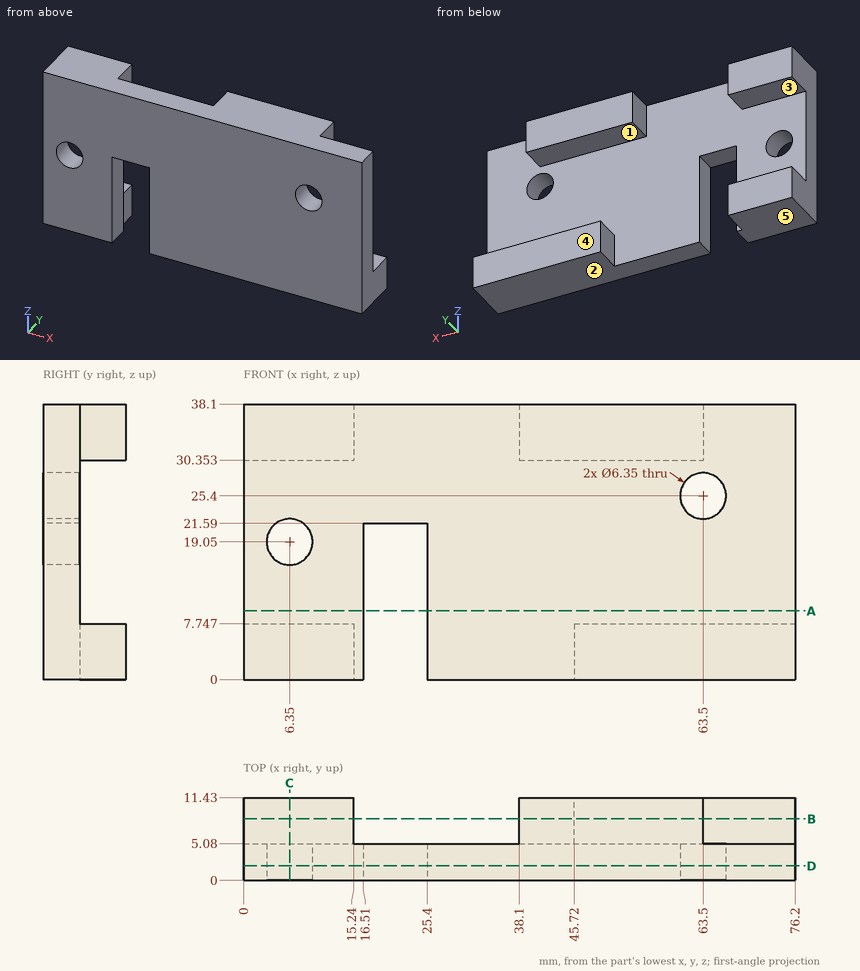
Answer from the drawing. Dimensions are ordinates in mm from the lowest x, y and z of the part. A direction names the side the tool comes from. Give positions to 0.01 mm unless a question says otherwise; leave off trailing zeros. Write each loop counter-clockwise with the first axis right and the second up, starting at its lowest first coordinate (ties: lowest second). Pieces come first, ordered by that corner, then holes. Notation, with made-up numbers: (53.25, 12) -> (62.25, 12) arc R22 ccw to (62.25, 46) -> close; hole circle Ø5 at (-23, 31.5). An arc over 180 degrees is marked (long way). Use a Markdown table: item, result.
(1) Determine the mould class of the marked faces 3, 4 and 5 for opening direction Z: released by +Z, released by -Z, zero draft, split by the parting line, or undercut.
Return value:
| item | result |
|---|---|
| face 3 | undercut |
| face 4 | zero draft |
| face 5 | released by -Z |
(2) Section A-A, the plane z = 9.5 is taken. Determine the outline of the cut face in (x, y), then the cut area to 3 significant figures.
Return value:
| item | result |
|---|---|
| outline | (0, 0) -> (16.51, 0) -> (16.51, 5.08) -> (0, 5.08) -> close; (25.4, 0) -> (76.2, 0) -> (76.2, 5.08) -> (25.4, 5.08) -> close |
| area | 342 mm2 |
(3) Find the intervals of material crossed by probe 1 along Z at (x, y) = (6.35, 1.3) (3 decimals); probe 2 along Z at (x, y) = (56.5, 8.75); probe 3 along X at (y, z) = (4.75, 7.5), in increasing order. Write a range as from..to.
Return value:
| item | result |
|---|---|
| probe 1 | 0..15.875, 22.225..38.1 |
| probe 2 | 0..7.75, 30.35..38.1 |
| probe 3 | 0..16.51, 25.4..76.2 |
(4) Flat-ended cylindrical pins translate along their axes: P1, Ø12, axis at x = 7.5, z = 19.5, coming from the +Y side; P2, Ø3, axis at y = 9, z = 35.5, coming from the +X side. Find the tip coordinate at first contact, or state that the pin passes through.
Return value:
| item | result |
|---|---|
| P1 | y = 5.08 |
| P2 | x = 63.5 |
(5) For the marked faces 1 and 2, determine the directions among +Z, -Z, +X, -X, +Y, -Y from which every point of the face is accessible in a straight line to the end or side of a thin tool.
Return value:
| item | result |
|---|---|
| face 1 | +X, -X, +Y |
| face 2 | -Z, +X, -X, +Y, -Y |
(6) Section D-D, the plane y = 2 is taken. Determine the outline of the cut face in (x, z) (3 decimals).
Return value:
| item | result |
|---|---|
| outline | (0, 0) -> (16.51, 0) -> (16.51, 21.59) -> (25.4, 21.59) -> (25.4, 0) -> (76.2, 0) -> (76.2, 38.1) -> (0, 38.1) -> close; hole circle Ø6.35 at (6.35, 19.05); hole circle Ø6.35 at (63.5, 25.4) |
(7) Section C-C, the plane x = 6.35 is taken. Determine the outline of the cut face in (y, z) (3 decimals).
Return value:
| item | result |
|---|---|
| outline | (0, 0) -> (11.43, 0) -> (11.43, 7.747) -> (5.08, 7.747) -> (5.08, 15.875) -> (0, 15.875) -> close; (0, 22.225) -> (5.08, 22.225) -> (5.08, 30.353) -> (11.43, 30.353) -> (11.43, 38.1) -> (0, 38.1) -> close |
(8) Section B-B, the plane y = 8.5 is taken. Determine the outline of the cut face in (x, z).
Return value:
| item | result |
|---|---|
| outline | (0, 0) -> (15.24, 0) -> (15.24, 7.75) -> (0, 7.75) -> close; (0, 30.35) -> (15.24, 30.35) -> (15.24, 38.1) -> (0, 38.1) -> close; (38.1, 30.35) -> (63.5, 30.35) -> (63.5, 38.1) -> (38.1, 38.1) -> close; (45.72, 0) -> (76.2, 0) -> (76.2, 7.75) -> (45.72, 7.75) -> close |
